```python
from build123d import *

# Parameters (mm, degrees)
SKETCH1_W           = 12
SKETCH1_H           = 31
SKETCH1_R           = 2.5
BOSS_EXTRUDE1_DEPTH = 1.12
SKETCH2_R           = 1.63
BOSS_EXTRUDE2_DEPTH = 31


with BuildPart() as part:
    # Sketch1 → Boss-Extrude1 (new body)
    with BuildSketch(Plane(origin=(0, 0, 0), x_dir=(1, 0, 0), z_dir=(0, 1, 0))):
        Rectangle(SKETCH1_W, SKETCH1_H)
        with Locations((0, 10)):
            Circle(SKETCH1_R, mode=Mode.SUBTRACT)
        with Locations((0, -10)):
            Circle(SKETCH1_R, mode=Mode.SUBTRACT)
    extrude(amount=BOSS_EXTRUDE1_DEPTH)

    # Sketch2 → Boss-Extrude2 (add)
    with BuildSketch(Plane.XY.offset(15.5)):
        with BuildLine():
            Line((-6, 1.12), (-6.535141088, 1.12))
            ThreePointArc((-6.535141088, 1.12), (-9.990967365, 5.204078238), (-8.75, 0))
            Line((-8.75, 0), (-6, 0))
            Line((-6, 0), (-6, 1.12))
        make_face()
        with Locations((-8.75, 2.75)):
            Circle(SKETCH2_R, mode=Mode.SUBTRACT)
    extrude(amount=-BOSS_EXTRUDE2_DEPTH)


solid = part.part
```
Input: part model. Units: mm. Frame: model coordinates. Give positions to 0.01 mm unless a question says otherwise; leave off trailing zeros. Order: outer loops, then holes, each group sorted by start corner. A loop starts at its lowest first (then second) coordinate and runs counter-clockwise, first axis right, second up. Notation, with made-up numbers: M -3,5 L 3,5 A24 ccw 3,23 Z; hole C 57.5,-9 d7. An arc over 180 degrees is marked long. One line per question, with ' | ' between items. Start each with the question number.
1. Section query B-B (y = 2.75). Return the cut outline in (x, z), and give its area (3 significant figures).
2. Section query C-C (x = 3.25). Return the cut outline in (y, z), and give its area (3 significant figures).
3. First-contact query: pin 1 Ø2 at (y, z) = (3.5, 7) entering from +X; pin 2 Ø6 at (x, z) = (0, -10) entering from +Y. Flat tips, straight axial feed; report the tip coordinate or a pass-through.
4. Pull-direction query (Z, two-part tool) for faces 1 (the face through (-4.82, 0.96, 15.5)), 2 (the face through (6, 0.6, 0.2)), 3 (the face through (-0.54, 0.55, -7.56)); classes: released by +Z, released by -Z, zero draft, split by the parting line, or undercut.
5. Material intervals for probe 1 along Z at (x, y) = (0, 0.75); probe 2 along Z at (x, y) = (-1.75, 0.5); probe 3 along Y at (x, z) = (-8.75, -1.5), sorted ascending. Write a range as [from, to].
6. Section query A-A (z = -10). Return the cut outline in (x, y).
7. Section query D-D (y = 0.45). Return the cut outline in (x, z), and give its area (3 significant figures).
Here are the results:
1) outline: M -11.5,-15.5 L -10.38,-15.5 L -10.38,15.5 L -11.5,15.5 Z; M -7.12,-15.5 L -6,-15.5 L -6,15.5 L -7.12,15.5 Z | area: 69.4 mm²
2) outline: M 0,-15.5 L 1.12,-15.5 L 1.12,15.5 L 0,15.5 Z | area: 34.7 mm²
3) pin 1: x = -6 | pin 2: y = 1.12
4) face 1: released by +Z | face 2: zero draft | face 3: undercut
5) probe 1: [-15.5, -12.5], [-7.5, 7.5], [12.5, 15.5] | probe 2: [-15.5, -11.79], [-8.21, 8.21], [11.79, 15.5] | probe 3: [0, 1.12], [4.38, 5.5]
6) outline: M -8.75,0 L -2.5,0 L -2.5,1.12 L -6.54,1.12 A2.75 ccw long Z; M 2.5,0 L 6,0 L 6,1.12 L 2.5,1.12 Z; hole C -8.75,2.75 d3.26
7) outline: M -10.26,-15.5 L 6,-15.5 L 6,15.5 L -10.26,15.5 Z; hole C 0,-10 d5; hole C 0,10 d5 | area: 465 mm²
